Model file for the job. Use its own axes, mm. A direction names the side the tool comes from. Coordinates: 2 decimals unless noted, no trailing zeros. Order: outer loops, then holes, each group sorted by start corner. A loop starts at its lowest first (then second) coordinate and runs counter-clockwise, first axis right, second up. Notation, with made-up numbers: (40, -2.5) -> (86, -2.5) arc R19 ccw to (86, 8.5) -> close; hole circle Ø10 at (-38, 56). An arc over 180 degrees is marked (long way). Return JSON: item names as keys, results as strings. Group by question number.
1) Probe line 1 (Z direction, x = 0, y = -21); line 2 (Z direction, x = 0, y = -35.6); line 3 (X direction, y = -6, z = 7.5). List the from-to ranges inside material, lowest first.
2) Cut at C-C (z = -3.5). Write the cut outline in (x, y), and give its area (3 significant figures).
3) Which spindle directions (+Z, -Z, +X, -X, +Y, -Y) get a long thin tool onto all of the face, cutting with end or side? Do faces 5 (the flat face through (4, -32.512, -12.4)), 6 (the flat face through (-31, -9, 31.75)), 7 (the cylindrical face through (102.333, -8.891, 0.329)). Say none if no direction does.
4) Flat gauge pins, fed straight in: pin 1 (10 mm diameter, centred on y = -26.5, z = 22, fed in from +X); pin 2 (10 mm diameter, centred on y = -14.5, z = 20, fed in from +X); pin 3 (5.5 mm diameter, centred on x = 72.5, y = -10.5, fed in from -Z); pin 4 (15 mm diameter, centred on x = -61.98, z = 0, fed in from -Y). Where does each tip first touch, or does it go through?
5) Pull direction X, two halves, no side cores. Call faces 1 (the flat face through (14, -37.592, -14)), 2 (the flat face through (73, -9, 14.953)), 3 (the cylindrical face through (-31.742, -27.805, 0.698)), 4 (the cylindrical face through (118.33, -8.89, -0.68)): +X half, -X half, draft (parallel to the pull), parting line (faces both ways), or undercut.
6) Cut at D-D (x = 100). Write the cut outline in (y, z).
7) Cut at B-B (y = -13). Write the cut outline in (x, z) (3 decimals).
from build123d import *

# Parameters (mm, degrees)
F0_R     = 9.525
F1_DEPTH = 18.288
F0_R_2   = 19.05
F2_DEPTH = 37.592
F3_DEPTH = 18.034
F0_R_3   = 12.7
F5_DEPTH = 32.512


# Not quite as in the source:
# - the program builds the solid bodies; features that only make, move or delete a surface that nothing else refers to are left out


with BuildPart() as f1:
    # F0 (on Front) → F1 (new body)
    with BuildSketch(Plane.XZ):
        with BuildLine():
            ThreePointArc((0, -31.75), (-31.75, 0), (0, 31.75))
            Line((0, 31.75), (-61.9795769453, 31.75))
            ThreePointArc((-61.9795769453, 31.75), (-93.7295769453, 0), (-61.9795769453, -31.75))
            Line((-61.9795769453, -31.75), (0, -31.75))
        make_face()
        with Locations((-61.9795769453, 0)):
            Circle(F0_R, mode=Mode.SUBTRACT)
    extrude(amount=F1_DEPTH)

    # F0 (on Front) → F2 (join)
    with BuildSketch(Plane.XZ):
        with BuildLine():
            Line((0.5778842542, 31.7447405059), (0, 31.75))
            ThreePointArc((0, 31.75), (-31.75, 0), (0, -31.75))
            Line((0, -31.75), (0.5778842542, -31.7447405059))
            ThreePointArc((0.5778842542, -31.7447405059), (22.6540319267, -22.2453891282), (31.75, 0))
            ThreePointArc((31.75, 0), (22.6540319267, 22.2453891282), (0.5778842542, 31.7447405059))
        make_face()
        Circle(F0_R_2, mode=Mode.SUBTRACT)
    extrude(amount=F2_DEPTH)

    # F0 (on Front) → F3 (join)
    with BuildSketch(Plane.XZ):
        with BuildLine():
            Line((87.3840512359, 30.9546921229), (0.5778842542, 31.7447405059))
            ThreePointArc((0.5778842542, 31.7447405059), (22.6540319267, 22.2453891282), (31.75, 0))
            ThreePointArc((31.75, 0), (22.6540319267, -22.2453891282), (0.5778842542, -31.7447405059))
            Line((0.5778842542, -31.7447405059), (87.3840512359, -30.9546921229))
            ThreePointArc((87.3840512359, -30.9546921229), (118.3387433588, 0), (87.3840512359, 30.9546921229))
        make_face()
        with BuildLine():
            ThreePointArc((59.4440512359, -14.9526921229), (44.491359113, 0), (59.4440512359, 14.9526921229))
            Line((59.4440512359, 14.9526921229), (87.3840512359, 14.9526921229))
            ThreePointArc((87.3840512359, 14.9526921229), (102.3367433588, 0), (87.3840512359, -14.9526921229))
            Line((87.3840512359, -14.9526921229), (59.4440512359, -14.9526921229))
        make_face(mode=Mode.SUBTRACT)
    extrude(amount=F3_DEPTH)

    # F0 (on Front) → F5 (join)
    with BuildSketch(Plane.XZ):
        Circle(F0_R_2)
        Circle(F0_R_3, mode=Mode.SUBTRACT)
    extrude(amount=F5_DEPTH)


solid = f1.part
Answers below:
{
 "1": {"line 1": "z = -31.75 to -12.7, 12.7 to 31.75", "line 2": "z = -31.75 to -19.05, 19.05 to 31.75", "line 3": "x = -92.83 to -67.85, -56.11 to -10.25, 10.25 to 46.51, 100.32 to 117.42"},
 "2": {"outline": "(-93.54, -18.29) -> (-70.84, -18.29) -> (-70.84, 0) -> (-93.54, 0) -> close; (-53.12, -18.29) -> (-31.56, -18.29) -> (-31.56, -37.59) -> (-18.73, -37.59) -> (-18.73, -32.51) -> (-12.21, -32.51) -> (-12.21, 0) -> (-53.12, 0) -> close; (12.21, -32.51) -> (18.73, -32.51) -> (18.73, -37.59) -> (31.56, -37.59) -> (31.56, -18.03) -> (44.91, -18.03) -> (44.91, 0) -> (12.21, 0) -> close; (101.92, -18.03) -> (118.14, -18.03) -> (118.14, 0) -> (101.92, 0) -> close", "area": "2,730 mm^2"},
 "3": {"face 5": "-Y", "face 6": "+Z, +X, -X, +Y, -Y", "face 7": "+Y, -Y"},
 "4": {"pin 1": "stops at x = 26.82", "pin 2": "stops at x = 114.46", "pin 3": "stops at z = -31.12", "pin 4": "passes through"},
 "5": {"face 1": "draft", "face 2": "undercut", "face 3": "-X half", "face 4": "+X half"},
 "6": {"outline": "(-18.03, -28.27) -> (0, -28.27) -> (0, -8.03) -> (-18.03, -8.03) -> close; (-18.03, 8.03) -> (0, 8.03) -> (0, 28.27) -> (-18.03, 28.27) -> close"},
 "7": {"outline": "(-61.98, -31.75) -> (0, -31.75) -> (87.384, -30.955) arc R30.955 ccw to (87.384, 30.955) -> (0, 31.75) -> (-61.98, 31.75) arc R31.75 ccw to start; hole circle Ø19.05 at (-61.98, 0); hole circle Ø25.4 at (0, 0); hole (59.444, -14.953) -> (87.384, -14.953) arc R14.953 ccw to (87.384, 14.953) -> (59.444, 14.953) arc R14.953 ccw to start"}
}
